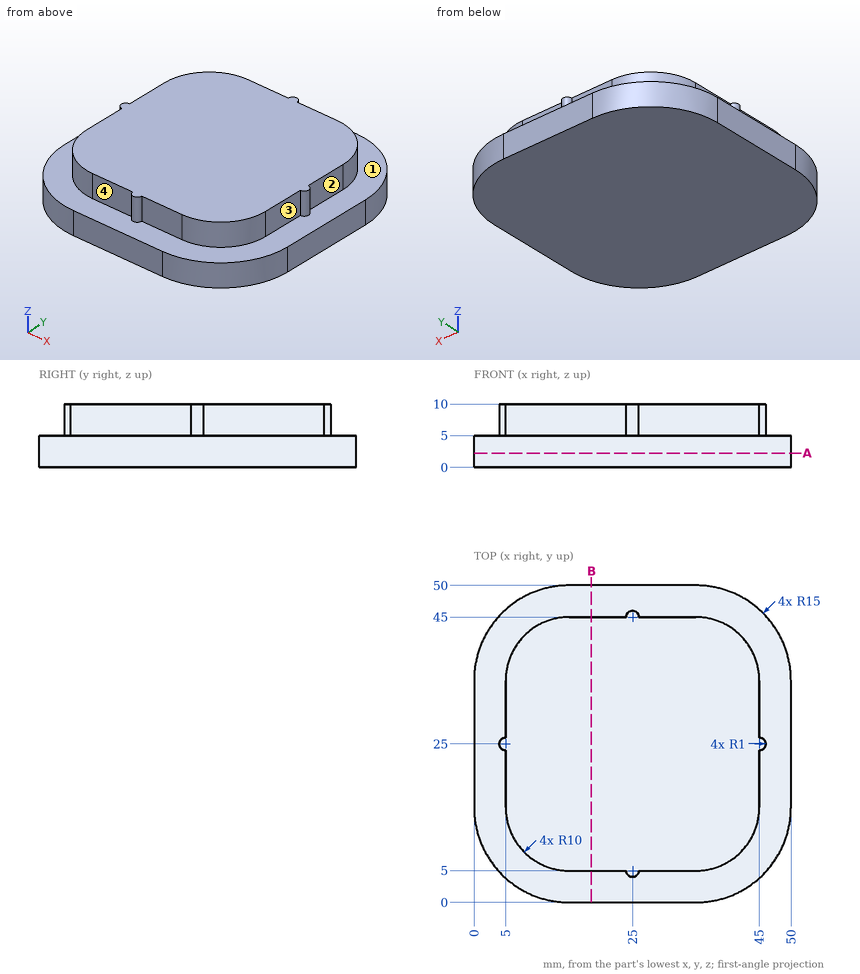
Verification items for this drawing (mm, ordinates from the low corner). A direction names the side the tool comes from. Give positions to 0.01 mm unless a question says otherwise; leave off trailing zeros. Loops run counter-clockwise (first coordinate to the right, second up) from the corner with the lowest first, then second, coordinate; pieces in that order, holes last.
1. Go/stop test with flat-tipped pins: P1, Ø1.5, axis at y = 28.5, z = 8.5, coming from the -X side; P2, Ø1.5, axis at y = 13.5, z = 8, coming from the +X side; P3, Ø2.5, axis at x = 18.5, z = 8, coming from the -Y side. Record where each tip stops, or that it passes through.
Derived:
P1: stops at x = 5
P2: stops at x = 44.97
P3: stops at y = 5
2. Tool access check on the marked faces 1, 2, 3 and 4. Record the directions out of +Z, -Z, +X, -X, +Y, -Y that give a thin tool (end or side, any length) a straight path to the whole face; none if there is none.
Derived:
face 1: +Z
face 2: +Z, +X, +Y
face 3: +Z, +X, -Y
face 4: +Z, -X, -Y
3. Cross-section at B-B on x = 18.5. Record the cut outline in (y, z), and give its area (3 significant figures).
Derived:
outline: (0, 0) - (50, 0) - (50, 5) - (45, 5) - (45, 10) - (5, 10) - (5, 5) - (0, 5) - close
area: 450 mm2
4. Material ranges on probe 1 along Y at (x, z) = (20.5, 8.25); probe 2 along Z at (x, y) = (11, 45), recorded low to high.
Derived:
probe 1: y = 5 to 45
probe 2: z = 0 to 5
5. Cross-section at A-A on z = 2.25. Record the cut outline in (x, y), and give its area (3 significant figures).
Derived:
outline: (0, 15) arc R15 ccw to (15, 0) - (35, 0) arc R15 ccw to (50, 15) - (50, 35) arc R15 ccw to (35, 50) - (15, 50) arc R15 ccw to (0, 35) - close
area: 2,310 mm2
